Can you work these out from the model? Positions are in its coordinate system, mm. Give positions to 0.01 mm unless a question says otherwise; leave off trailing zeros. Loops run counter-clockwise (first coordinate to the right, second up) from the corner with the lowest first, then second, coordinate; pieces in that order, holes last. Notation, with made-up numbers: (-30.5, 58) - (-15.5, 58) arc R26 cw to (-15.5, 78) - close; hole circle Ø8 at (81, 85.25). An arc over 180 degrees is marked (long way). Answer as a JSON object with one key per item and string values.
```python
from build123d import *

# Parameters (mm, degrees)
ESQUISSE1_W             = 15
ESQUISSE1_H             = 15
BOSS_EXTRU_1_DEPTH      = 50
ESQUISSE2_R             = 2.25
ENL_V_MAT_EXTRU_1_DEPTH = 55.313902456
ESQUISSE3_R             = 2.25
ENL_V_MAT_EXTRU_2_DEPTH = 55.313902456


with BuildPart() as part:
    # Esquisse1 → Boss.-Extru.1 (new body)
    with BuildSketch(Plane.XY):
        with Locations((7.5, 7.5)):
            Rectangle(ESQUISSE1_W, ESQUISSE1_H)
    extrude(amount=BOSS_EXTRU_1_DEPTH)

    # Esquisse2 → Enlèv. mat.-Extru.1 (cut, through all)
    with BuildSketch(Plane(origin=(0, 15, 0), x_dir=(1, 0, 0), z_dir=(0, 1, 0))):
        with Locations(Location((7.5, -44.5, 0), (0, 0, 270))):
            Circle(ESQUISSE2_R)
        with Locations(Location((7.5, -5.5, 0), (0, 0, 90))):
            Circle(ESQUISSE2_R)
    extrude(amount=-ENL_V_MAT_EXTRU_1_DEPTH, mode=Mode.SUBTRACT)

    # Esquisse3 → Enlèv. mat.-Extru.2 (cut, through all)
    with BuildSketch(Plane.ZY):
        with Locations((23.05, 7.5)):
            Circle(ESQUISSE3_R)
        with Locations((35.05, 7.5)):
            Circle(ESQUISSE3_R)
        with Locations(Location((11.05, 7.5, 0), (0, 0, 180))):
            Circle(ESQUISSE3_R)
    extrude(amount=-ENL_V_MAT_EXTRU_2_DEPTH, mode=Mode.SUBTRACT)


solid = part.part
```
1) I need wall thicknesses on L1, parallel to X at y = 12, z = 5.5; L2, parallel to Z at x = 2, y = 6. Which ranges of each line are inside material? Lowest first, please.
Check sheet entries:
{"L1": "0 to 5.25, 9.75 to 15", "L2": "0 to 9.37, 12.73 to 21.37, 24.73 to 33.37, 36.73 to 50"}
2) Imagine slicing it at B-B on z = 23.05. Write out the boundary of the cut face in (x, y).
Check sheet entries:
{"outline": "(0, 0) - (15, 0) - (15, 5.25) - (0, 5.25) - close; (0, 9.75) - (15, 9.75) - (15, 15) - (0, 15) - close"}
3) Imagine slicing it at D-D on x = 1. Write out the boundary of the cut face in (y, z).
Check sheet entries:
{"outline": "(0, 0) - (15, 0) - (15, 50) - (0, 50) - close; hole circle Ø4.5 at (7.5, 11.05); hole circle Ø4.5 at (7.5, 23.05); hole circle Ø4.5 at (7.5, 35.05)"}
4) Imagine slicing it at A-A on y = 7.5. Write out the boundary of the cut face in (x, z).
Check sheet entries:
{"outline": "(0, 0) - (15, 0) - (15, 8.8) - (0, 8.8) - close; (0, 13.3) - (15, 13.3) - (15, 20.8) - (0, 20.8) - close; (0, 25.3) - (15, 25.3) - (15, 32.8) - (0, 32.8) - close; (0, 37.3) - (15, 37.3) - (15, 50) - (0, 50) - close; hole circle Ø4.5 at (7.5, 5.5); hole circle Ø4.5 at (7.5, 44.5)"}
5) If we mould it in two halves opening along X, with no side actions, what happens to faces 1 (the cylindrical face through (7.395, 7.599, 32.802)), 2 (the cylindrical face through (5.603, 7.605, 4.29)), 3 (the flat face through (15, 6, 25))? For each: released by +X, released by -X, zero draft, split by the parting line, or undercut.
Check sheet entries:
{"face 1": "zero draft", "face 2": "undercut", "face 3": "released by +X"}
6) I'm going to push a flat-ended pin straight in: P1, Ø2.5, axis at y = 7.5, z = 23.05, coming from the -X side. Where does the tip first touch, or does it pass through?
Check sheet entries:
{"P1": "through"}
7) Imagine slicing it at C-C on x = 7.5. Write out the boundary of the cut face in (y, z), and give its area (3 significant figures).
Check sheet entries:
{"outline": "(0, 0) - (15, 0) - (15, 3.25) - (0, 3.25) - close; (0, 7.75) - (15, 7.75) - (15, 42.25) - (0, 42.25) - close; (0, 46.75) - (15, 46.75) - (15, 50) - (0, 50) - close; hole circle Ø4.5 at (7.5, 11.05); hole circle Ø4.5 at (7.5, 23.05); hole circle Ø4.5 at (7.5, 35.05)", "area": "567 mm2"}
